from build123d import *

# Parameters (mm, degrees)
F0_R      = 67
F1_DEPTH  = 5
F2_R      = 64.375
F2_R_2    = 62.625
F3_DEPTH  = 3
F2_R_3    = 58.875
F4_DEPTH  = 2
F5_R      = 4.75
F5_R_2    = 5.75
F5_R_3    = 2.1
F6_DEPTH  = 25
F7_R      = 5.75
F7_R_2    = 6.75
F8_DEPTH  = 0.5
F8_TAPER  = -3
F10_DEPTH = 3
F10_TAPER = -3
F11_R     = 6.75
F12_DEPTH = 1
F13_W     = 5
F13_H     = 12
F14_DEPTH = 1.5
F15_COUNT = 6
F15_ANGLE = 150
F16_COUNT = 6
F16_ANGLE = 150


with BuildPart() as f1:
    # F0 (on Front) → F1 (new body)
    with BuildSketch(Plane.XZ):
        Circle(F0_R)
    extrude(amount=F1_DEPTH)

    # F2 (on face) → F3 (join)
    with BuildSketch(Plane.XZ.offset(5)):
        Circle(F2_R)
        Circle(F2_R_2, mode=Mode.SUBTRACT)
    extrude(amount=F3_DEPTH)

    # F2 (on face) → F4 (cut)
    with BuildSketch(Plane.XZ.offset(5)):
        Circle(F2_R_2)
        Circle(F2_R_3, mode=Mode.SUBTRACT)
    extrude(amount=-F4_DEPTH, mode=Mode.SUBTRACT)

    # F5 (on face) → F6 (cut)
    with BuildSketch(Plane.XZ.offset(5)):
        Circle(F5_R)
        with Locations((0, 18.75)):
            Circle(F5_R_2)
        with Locations((0, 46.25)):
            Circle(F5_R_2)
        with Locations((17.5, -8)):
            Circle(F5_R_3)
        with Locations((-17.5, -8)):
            Circle(F5_R_3)
    extrude(amount=-F6_DEPTH, mode=Mode.SUBTRACT)

    # F7 (on face) → F8 (cut)
    with BuildSketch(Plane.XZ.offset(5)):
        Circle(F7_R)
        with Locations((0, 18.75)):
            Circle(F7_R_2)
        with Locations((0, 46.25)):
            Circle(F7_R_2)
    extrude(amount=-F8_DEPTH, taper=F8_TAPER, mode=Mode.SUBTRACT)

    # F9 (on face) → F10 (cut)
    with BuildSketch(Plane.XZ.offset(5)):
        Polygon((21.25, -10.1650635095), (21.25, -5.8349364905), (17.5, -3.6698729811), (13.75, -5.8349364905), (13.75, -10.1650635095), (17.5, -12.3301270189), align=None)
        Polygon((-17.5, -3.6698729811), (-21.25, -5.8349364905), (-21.25, -10.1650635095), (-17.5, -12.3301270189), (-13.75, -10.1650635095), (-13.75, -5.8349364905), align=None)
    extrude(amount=-F10_DEPTH, taper=F10_TAPER, mode=Mode.SUBTRACT)

    # F11 (on Front) → F12 (cut)
    with BuildSketch(Plane.XZ):
        with Locations((0, 46.25)):
            Circle(F11_R)
        with Locations((0, 18.75)):
            Circle(F11_R)
    extrude(amount=F12_DEPTH, mode=Mode.SUBTRACT)

    # F13 (on face) → F14 (join)
    with BuildSketch(Plane.XZ.offset(5)):
        with Locations((0, -50)):
            Rectangle(F13_W, F13_H)
    f14 = extrude(amount=F14_DEPTH)

    # F15: F14 ×6 about axis
    f15_axis = Axis((0, -5, 0), (0, -1, 0))
    for i in range(1, F15_COUNT):
        add(f14.rotate(f15_axis, i * F15_ANGLE / (F15_COUNT - 1)))

    # F16: F14 ×6 about axis
    f16_axis = Axis((0, -5, 0), (0, 1, 0))
    for i in range(1, F16_COUNT):
        add(f14.rotate(f16_axis, i * F16_ANGLE / (F16_COUNT - 1)))


solid = f1.part
Verification items for the finished model (mm, model axes). A direction names the side the tool comes from. Round coordinates to 2 decimals unless told otherwise and drop trailing zeros. Loops run counter-clockwise (first coordinate to the right, second up) from the corner with the lowest first, then second, coordinate; pieces in that order, holes last. Notation, with made-up numbers: (69, 89) - (88, 89) arc R13 cw to (88, 98) - close; hole circle Ø10 at (76.5, -32.5). An arc over 180 degrees is marked (long way). Answer in a Markdown table with one row per item. Add a question column.
Q1. Section check B-B on x = -53. Enter the section's corners in (y, z).
Q2. Release check for a two-part mould opening along X. For faces 1 (the face through (-13.955, -6.479, -62.844)), 2 (the face through (-35, -5, 55)), 3 (the face through (-1.246, -2.774, 13.137)) record: pulls with the +X half, pulls with the -X half, needs draft (parallel to the pull), parting line crosses it, or undercut.
Q3. Material ranges on line 1 (Z direction, x = 0, y = -3.65) (3 decimals); line 2 (Z direction, x = -30, y = -4.25); line 3 (Z direction, x = -49, y = -4), recorded low to high.
Q4. Section check C-C on x = 10. Enter the section's corners in (y, z).
Q5. Tool access check on faces 4 (the face through (-1, 0, -14)), 5 (the face through (25, -6.5, -43)). Record the directions out of +Z, -Z, +X, -X, +Y, -Y that give a thin tool (end or side, any length) a straight path to the whole face; none if there is none.
Q6. Section check A-A on z = -28.5. Enter the section's corners in (x, y), plus the area to 3 significant figures.
Q7. Gauge pin test, flat ends, axial feed: pin 1 (8.5 mm diameter, centred on x = 16.5, z = -7.5, fed in from -Y); pin 2 (1.5 mm diameter, centred on y = -1.5, z = -3, fed in from +X); pin 3 (2 mm diameter, centred on y = -4.5, z = -30.5, fed in from -X). Record the tip position at first contact, or that the pin passes through.
Found:
| question | item | result |
|---|---|---|
| 1 | outline | (-8, -36.54) - (-5, -36.54) - (-5, -40.99) - (0, -40.99) - (0, 40.99) - (-5, 40.99) - (-5, 36.54) - (-8, 36.54) - (-8, 33.36) - (-3, 33.36) - (-3, 25.64) - (-5, 25.64) - (-5, 2.5) - (-6.5, 2.5) - (-6.5, -2.5) - (-5, -2.5) - (-5, -25.64) - (-3, -25.64) - (-3, -33.36) - (-8, -33.36) - close |
| 2 | face 1 | parting line crosses it |
| 2 | face 2 | needs draft |
| 2 | face 3 | undercut |
| 3 | line 1 | z = -67 to -62.625, -58.875 to -4.75, 4.75 to 13, 24.5 to 40.5, 52 to 58.875, 62.625 to 67 |
| 3 | line 2 | z = -59.91 to -54.97, -50.66 to 50.66, 54.97 to 59.91 |
| 3 | line 3 | z = -45.69 to -39, -32.64 to 32.64, 39 to 45.69 |
| 4 | outline | (-8, -63.59) - (-5, -63.59) - (-5, -66.25) - (0, -66.25) - (0, 66.25) - (-5, 66.25) - (-5, 63.59) - (-8, 63.59) - (-8, 61.82) - (-3, 61.82) - (-3, 58.02) - (-5, 58.02) - (-5, -58.02) - (-3, -58.02) - (-3, -61.82) - (-8, -61.82) - close |
| 5 | face 4 | +Z, -Z, +X, -X, +Y |
| 5 | face 5 | -Y |
| 6 | outline | (-60.64, -5) - (-57.72, -5) - (-57.72, -8) - (-55.76, -8) - (-55.76, -3) - (-51.52, -3) - (-51.52, -5) - (-48.21, -5) - (-48.21, -6.5) - (-44.36, -6.5) - (-44.36, -5) - (44.36, -5) - (44.36, -6.5) - (48.21, -6.5) - (48.21, -5) - (51.52, -5) - (51.52, -3) - (55.76, -3) - (55.76, -8) - (57.72, -8) - (57.72, -5) - (60.64, -5) - (60.64, 0) - (-60.64, 0) - close |
| 6 | area | 613 mm² |
| 7 | pin 1 | stops at y = -5 |
| 7 | pin 2 | stops at x = 66.96 |
| 7 | pin 3 | stops at x = -60.16 |
